from build123d import *

# Parameters (mm, degrees)
SKETCH_1_W          = 500
SKETCH_1_H          = 250
EXTRUDE_1_DEPTH     = 3.6
SKETCH_2_W          = 50
SKETCH_2_H          = 4
CUT_EXTRUDE_1_DEPTH = 3.6
SKETCH_3_W          = 4
SKETCH_3_H          = 50
SKETCH_3_H_2        = 41.448480175
CUT_EXTRUDE_2_DEPTH = 3.6
SKETCH_4_R          = 2
CUT_EXTRUDE_3_DEPTH = 280.531679779
SKETCH_5_R          = 2
CUT_EXTRUDE_4_DEPTH = 10
SKETCH_7_R          = 2.5
CUT_EXTRUDE_5_DEPTH = 10
SKETCH_9_R          = 2.25
CUT_EXTRUDE_6_DEPTH = 280.531679779
SKETCH_10_R         = 2.5
CUT_EXTRUDE_7_DEPTH = 280.531679779


with BuildPart() as part:
    # 草图1 → 凸台-拉伸1 (new body)
    with BuildSketch(Plane.XY):
        Rectangle(SKETCH_1_W, SKETCH_1_H)
    extrude(amount=EXTRUDE_1_DEPTH)

    # 草图2 → 切除-拉伸1 (cut)
    with BuildSketch(Plane.XY.offset(3.6)):
        with Locations((0, 123)):
            Rectangle(SKETCH_2_W, SKETCH_2_H)
        with Locations((-110, 123)):
            Rectangle(SKETCH_2_W, SKETCH_2_H)
        with Locations((-210, 123)):
            Rectangle(SKETCH_2_W, SKETCH_2_H)
        with Locations((110, 123)):
            Rectangle(SKETCH_2_W, SKETCH_2_H)
        with Locations((210, 123)):
            Rectangle(SKETCH_2_W, SKETCH_2_H)
        with Locations((210, -123)):
            Rectangle(SKETCH_2_W, SKETCH_2_H)
        with Locations((110, -123)):
            Rectangle(SKETCH_2_W, SKETCH_2_H)
        with Locations((-210, -123)):
            Rectangle(SKETCH_2_W, SKETCH_2_H)
        with Locations((-110, -123)):
            Rectangle(SKETCH_2_W, SKETCH_2_H)
        with Locations((0, -123)):
            Rectangle(SKETCH_2_W, SKETCH_2_H)
    extrude(amount=-CUT_EXTRUDE_1_DEPTH, mode=Mode.SUBTRACT)

    # 草图3 → 切除-拉伸2 (cut)
    with BuildSketch(Plane.XY.offset(3.6)):
        with Locations((-248, 0)):
            Rectangle(SKETCH_3_W, SKETCH_3_H)
        with Locations((-248, 110)):
            Rectangle(SKETCH_3_W, SKETCH_3_H)
        with Locations((-248, -110)):
            Rectangle(SKETCH_3_W, SKETCH_3_H)
        with Locations((248, 4.275759912)):
            Rectangle(SKETCH_3_W, SKETCH_3_H_2)
        with Locations((248, -101.448480175)):
            Rectangle(SKETCH_3_W, SKETCH_3_H)
        with Locations((248, 110)):
            Rectangle(SKETCH_3_W, SKETCH_3_H)
    extrude(amount=-CUT_EXTRUDE_2_DEPTH, mode=Mode.SUBTRACT)

    # 草图4 → 切除-拉伸3 (cut, through all)
    with BuildSketch(Plane.XY.offset(3.6)):
        with Locations((80, 75)):
            Circle(SKETCH_4_R)
        with Locations((80, -52)):
            Circle(SKETCH_4_R)
        with Locations((80, 52)):
            Circle(SKETCH_4_R)
        with Locations((80, -75)):
            Circle(SKETCH_4_R)
    extrude(amount=-CUT_EXTRUDE_3_DEPTH, mode=Mode.SUBTRACT)

    # 草图5 → 切除-拉伸4 (cut)
    with BuildSketch(Plane.XY.offset(3.6)):
        with Locations((50, 75)):
            Circle(SKETCH_5_R)
        with Locations((50, 52)):
            Circle(SKETCH_5_R)
        with Locations((50, -52)):
            Circle(SKETCH_5_R)
        with Locations((50, -75)):
            Circle(SKETCH_5_R)
    extrude(amount=-CUT_EXTRUDE_4_DEPTH, mode=Mode.SUBTRACT)

    # 草图7 → 切除-拉伸5 (cut)
    with BuildSketch(Plane.XY.offset(3.6)):
        with Locations((161, -17.5)):
            Circle(SKETCH_7_R)
        with Locations((161, 17.5)):
            Circle(SKETCH_7_R)
    extrude(amount=-CUT_EXTRUDE_5_DEPTH, mode=Mode.SUBTRACT)

    # 草图9 → 切除-拉伸6 (cut, through all)
    with BuildSketch(Plane.XY.offset(3.6)):
        with Locations((70, 20)):
            Circle(SKETCH_9_R)
        with Locations((100, 20)):
            Circle(SKETCH_9_R)
        with Locations((70, -20)):
            Circle(SKETCH_9_R)
        with Locations((100, -20)):
            Circle(SKETCH_9_R)
    extrude(amount=-CUT_EXTRUDE_6_DEPTH, mode=Mode.SUBTRACT)

    # 草图10 → 切除-拉伸7 (cut, through all)
    with BuildSketch(Plane.XY.offset(3.6)):
        with Locations((-208, 110)):
            Circle(SKETCH_10_R)
        with Locations((-189, 110)):
            Circle(SKETCH_10_R)
        with Locations((-208, 80)):
            Circle(SKETCH_10_R)
        with Locations((-189, 80)):
            Circle(SKETCH_10_R)
        with Locations(Location((-189, -110, 0), (0, 0, 180))):
            Circle(SKETCH_10_R)
        with Locations(Location((-189, -80, 0), (0, 0, 180))):
            Circle(SKETCH_10_R)
        with Locations(Location((-208, -80, 0), (0, 0, 180))):
            Circle(SKETCH_10_R)
        with Locations(Location((-208, -110, 0), (0, 0, 180))):
            Circle(SKETCH_10_R)
        with Locations((149, 110)):
            Circle(SKETCH_10_R)
        with Locations((168, 110)):
            Circle(SKETCH_10_R)
        with Locations((149, 80)):
            Circle(SKETCH_10_R)
        with Locations((168, 80)):
            Circle(SKETCH_10_R)
        with Locations(Location((168, -110, 0), (0, 0, 180))):
            Circle(SKETCH_10_R)
        with Locations(Location((168, -80, 0), (0, 0, 180))):
            Circle(SKETCH_10_R)
        with Locations(Location((149, -80, 0), (0, 0, 180))):
            Circle(SKETCH_10_R)
        with Locations(Location((149, -110, 0), (0, 0, 180))):
            Circle(SKETCH_10_R)
    extrude(amount=-CUT_EXTRUDE_7_DEPTH, mode=Mode.SUBTRACT)


solid = part.part
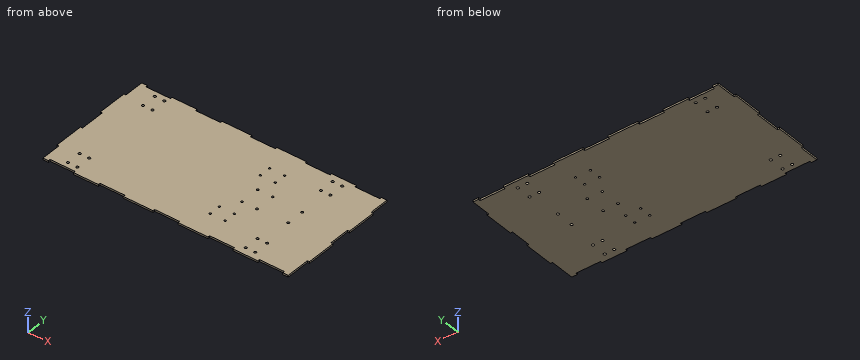
The listing builds one solid part. Answer for the finished solid, in the listing's coordinates (mm). Round coordinates to 2 decimals unless told otherwise and drop trailing zeros. Loops run counter-clockwise (first coordinate to the right, second up) from the corner with the lowest first, then second, coordinate; pieces in that order, holes last. Notation, with made-up numbers: M 52,1 L 57,1 A22 cw 57,14 Z; hole C 79,29.25 d5. An arc over 180 degrees is marked long. Write each question's results on one line, items separated by ' | '. Start each with the question number.
1) Find section B-B on z = 0.8. Count the separate pieces of the cut face and the enclosed holes in it, plus the area to 3 significant figures.
2) This flat-tipped pin is pushed along its axis until it touches: pin 1 (1.8 mm diameter, centred on x = -249, z = 1.5, fed in from +Y). Where does it stop, or does it pass through?
3) Find section A-A on x = 205. Write down the section's boundary in (y, z).
4) Straight lines are drawn through the part: probe 1 along Y at (x, z) = (-208, 1.95); probe 2 along Y at (x, z) = (149, 2.5); probe 3 along Y at (x, z) = (99.5, 2.25). For each, find the intervals that lie inside material, in ascending order.
Final values:
1) separate pieces: 1 | enclosed holes: 30 | area: 121,000 mm²
2) pin 1: y = 85
3) outline: M -121,0 L 121,0 L 121,3.6 L -121,3.6 Z
4) probe 1: -121 to -112.5, -107.5 to -82.5, -77.5 to 77.5, 82.5 to 107.5, 112.5 to 121 | probe 2: -125 to -112.5, -107.5 to -82.5, -77.5 to 77.5, 82.5 to 107.5, 112.5 to 125 | probe 3: -121 to -22.19, -17.81 to 17.81, 22.19 to 121
